Verification items for the finished model (mm, model axes). A direction names the side the tool comes from. Coordinates: 2 decimals unless noted, no trailing zeros. Order: outer loops, then holes, each group sorted by start corner. A loop starts at its lowest first (then second) coordinate and runs counter-clockwise, first axis right, second up. Notation, with made-up numbers: (-5.75, 1.5) - (28.25, 1.5) arc R23 cw to (28.25, 13.5) - close; hole circle Ø11 at (12, 48.25). An arc over 180 degrees is marked (long way). One line per question, with ' | ' between items. Start each with the question number.
from build123d import *

# Parameters (mm, degrees)
CROQUIS12_W           = 115
CROQUIS12_H           = 329.4
BRIDA_BASE2_DEPTH     = 2
CORTAR_EXTRUIR6_REACH = 217.801
CROQUIS27_R           = 2
CORTAR_EXTRUIR7_REACH = 217.801
CROQUIS28_R           = 7.5
CROQUIS29_W           = 16
CROQUIS29_H           = 35
CORTAR_EXTRUIR8_DEPTH = 216.801042861
REDONDEO1_R           = 6
REDONDEO2_R           = 2


# Sheet-metal steps are written as plain solids
with BuildPart() as part:
    # Croquis12 → Brida base2 (new body)
    with BuildSketch(Plane(origin=(0, 0, 0), x_dir=(1, 0, 0), z_dir=(0, 1, 0))):
        with Locations((0, -43.29)):
            Rectangle(CROQUIS12_W, CROQUIS12_H)
    extrude(amount=-BRIDA_BASE2_DEPTH)

    # Croquis27 → Cortar-Extruir6 (cut, up to next)
    with BuildSketch(Plane(origin=(0, 0, 0), x_dir=(1, 0, 0), z_dir=(0, 1, 0)), mode=Mode.PRIVATE) as cortar_extruir6_sk1:
        with Locations(Location((-53.5, -201.3, 0), (0, 0, 270))):
            Circle(CROQUIS27_R)
    cortar_extruir6_tool1 = extrude(cortar_extruir6_sk1.sketch, amount=-CORTAR_EXTRUIR6_REACH, mode=Mode.PRIVATE) & part.part
    # Croquis27 → Cortar-Extruir6 (cut, up to next)
    with BuildSketch(Plane(origin=(0, 0, 0), x_dir=(1, 0, 0), z_dir=(0, 1, 0)), mode=Mode.PRIVATE) as cortar_extruir6_sk2:
        with Locations(Location((-53.5, 78.26, 0), (0, 0, 270))):
            Circle(CROQUIS27_R)
    cortar_extruir6_tool2 = extrude(cortar_extruir6_sk2.sketch, amount=-CORTAR_EXTRUIR6_REACH, mode=Mode.PRIVATE) & part.part
    # Croquis27 → Cortar-Extruir6 (cut, up to next)
    with BuildSketch(Plane(origin=(0, 0, 0), x_dir=(1, 0, 0), z_dir=(0, 1, 0)), mode=Mode.PRIVATE) as cortar_extruir6_sk3:
        with Locations(Location((53.5, 78.26, 0), (0, 0, 90))):
            Circle(CROQUIS27_R)
    cortar_extruir6_tool3 = extrude(cortar_extruir6_sk3.sketch, amount=-CORTAR_EXTRUIR6_REACH, mode=Mode.PRIVATE) & part.part
    # Croquis27 → Cortar-Extruir6 (cut, up to next)
    with BuildSketch(Plane(origin=(0, 0, 0), x_dir=(1, 0, 0), z_dir=(0, 1, 0)), mode=Mode.PRIVATE) as cortar_extruir6_sk4:
        with Locations(Location((53.5, -201.3, 0), (0, 0, 90))):
            Circle(CROQUIS27_R)
    cortar_extruir6_tool4 = extrude(cortar_extruir6_sk4.sketch, amount=-CORTAR_EXTRUIR6_REACH, mode=Mode.PRIVATE) & part.part
    add(cortar_extruir6_tool1.solids().sort_by_distance((-53.5, 0, 201.3))[0], mode=Mode.SUBTRACT)
    add(cortar_extruir6_tool2.solids().sort_by_distance((-53.5, 0, -78.26))[0], mode=Mode.SUBTRACT)
    add(cortar_extruir6_tool3.solids().sort_by_distance((53.5, 0, -78.26))[0], mode=Mode.SUBTRACT)
    add(cortar_extruir6_tool4.solids().sort_by_distance((53.5, 0, 201.3))[0], mode=Mode.SUBTRACT)

    # Croquis28 → Cortar-Extruir7 (cut, up to next)
    with BuildSketch(Plane(origin=(0, 0, 0), x_dir=(1, 0, 0), z_dir=(0, 1, 0)), mode=Mode.PRIVATE) as cortar_extruir7_sk1:
        with Locations(Location((0, 96.25, 0), (0, 0, 270))):
            Circle(CROQUIS28_R)
    cortar_extruir7_tool1 = extrude(cortar_extruir7_sk1.sketch, amount=-CORTAR_EXTRUIR7_REACH, mode=Mode.PRIVATE) & part.part
    add(cortar_extruir7_tool1.solids().sort_by_distance((0, 0, -96.25))[0], mode=Mode.SUBTRACT)

    # Croquis29 → Cortar-Extruir8 (cut, through all)
    with BuildSketch(Plane(origin=(0, 0, 0), x_dir=(1, 0, 0), z_dir=(0, 1, 0))):
        with Locations((39, 103.91)):
            Rectangle(CROQUIS29_W, CROQUIS29_H)
    extrude(amount=-CORTAR_EXTRUIR8_DEPTH, mode=Mode.SUBTRACT)

    # Redondeo1
    redondeo1_edges = [part.edges().sort_by_distance(p)[0] for p in [
        (31, -1, -86.41),
        (47, -1, -86.41),
    ]]
    fillet(redondeo1_edges, radius=REDONDEO1_R)

    # Redondeo2
    redondeo2_edges = [part.edges().sort_by_distance(p)[0] for p in [
        (31, -1, -121.41),
        (47, -1, -121.41),
    ]]
    fillet(redondeo2_edges, radius=REDONDEO2_R)


solid = part.part
Item 1: Thickness scan on probe 1 along X at (y, z) = (-1.4, 201.3); probe 2 along Z at (x, y) = (53.5, -0.65); probe 3 along X at (y, z) = (-0.8, -96.25). Record the ranges inside material, lowest first. Write a range as from..to.
Item 2: Section check C-C (x = 0). Record the cut outline in (y, z), then the cut area to 3 significant figures.
Item 3: Set-up check for faces 1 (the cylindrical face through (32.711, -1.014, -88.214)), 2 (the flat face through (-1, -2, 41)): record each of +Z, -Z, +X, -X, +Y, -Y from which the full face is reachable in a straight line by a thin tool's end or side.
Item 4: Mould release check, pull along X, two halves, no side actions. Record for faces 3 (the cylindrical face through (2.253, -0.986, -89.096)), 4 (the flat face through (-1, 0, 41)): +X half, -X half, draft (parallel to the pull), parting line (faces both ways), or undercut.
Item 5: Section check B-B (z = -96.25). Record the cut outline in (x, y).
Item 6: Section check A-A (y = -1.15). Record the cut outline in (x, z).
Completed:
1) probe 1: x = -57.5..-55.5, -51.5..51.5, 55.5..57.5 | probe 2: z = -121.41..-80.26, -76.26..199.3, 203.3..207.99 | probe 3: x = -57.5..-7.5, 7.5..31, 47..57.5
2) outline: (-2, -121.41) - (0, -121.41) - (0, -103.75) - (-2, -103.75) - close; (-2, -88.75) - (0, -88.75) - (0, 207.99) - (-2, 207.99) - close | area: 629 mm^2
3) face 1: -Z, +Y, -Y | face 2: +Z, -Z, +X, -X, -Y
4) face 3: undercut | face 4: draft
5) outline: (-57.5, -2) - (-7.5, -2) - (-7.5, 0) - (-57.5, 0) - close; (7.5, -2) - (31, -2) - (31, 0) - (7.5, 0) - close; (47, -2) - (57.5, -2) - (57.5, 0) - (47, 0) - close
6) outline: (-57.5, -121.41) - (29, -121.41) arc R2 ccw to (31, -119.41) - (31, -92.41) arc R6 cw to (37, -86.41) - (41, -86.41) arc R6 cw to (47, -92.41) - (47, -119.41) arc R2 ccw to (49, -121.41) - (57.5, -121.41) - (57.5, 207.99) - (-57.5, 207.99) - close; hole circle Ø4 at (-53.5, -78.26); hole circle Ø4 at (-53.5, 201.3); hole circle Ø15 at (0, -96.25); hole circle Ø4 at (53.5, -78.26); hole circle Ø4 at (53.5, 201.3)
